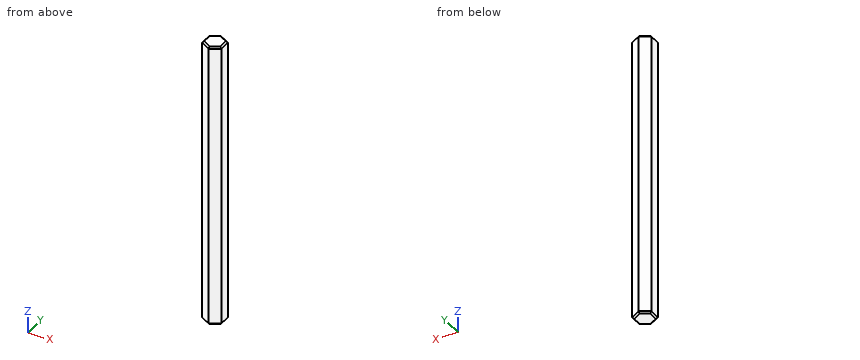
```python
from build123d import *

# Parameters (mm, degrees)
BOSS_EXTRUDE1_DEPTH = 75
CHAMFER1_SIZE       = 0.4


with BuildPart() as part:
    # Sketch1 → Boss-Extrude1 (new body)
    with BuildSketch(Plane.XY.offset(75)):
        Polygon((0, -2.886751346), (2.5, -1.443375673), (2.5, 1.443375673), (0, 2.886751346), (-2.5, 1.443375673), (-2.5, -1.443375673), align=None)
    extrude(amount=-BOSS_EXTRUDE1_DEPTH)

    # Chamfer1
    chamfer1_edges = [part.edges().sort_by_distance(p)[0] for p in [
        (2.5, 0, 0),
        (1.25, 2.165063509, 0),
        (-1.25, 2.165063509, 0),
        (-2.5, 0, 0),
        (-1.25, -2.165063509, 0),
        (-2.5, 0, 75),
        (-1.25, 2.165063509, 75),
        (1.25, 2.165063509, 75),
        (1.25, -2.165063509, 0),
        (2.5, 0, 75),
        (1.25, -2.165063509, 75),
        (-1.25, -2.165063509, 75),
    ]]
    chamfer(chamfer1_edges, length=CHAMFER1_SIZE)


solid = part.part
```
Work out the finished part from the listing and answer in its coordinate system (mm). Round coordinates to 2 decimals unless told otherwise and drop trailing zeros. Loops run counter-clockwise (first coordinate to the right, second up) from the corner with the lowest first, then second, coordinate; pieces in that order, holes last. Notation, with made-up numbers: M -28,37.25 L 14,37.25 A18 ccw 14,66.25 Z; hole C 46.5,67 d5. An arc over 180 degrees is marked long. Use CSV: the item, a comma, the result in double quotes.
Q1. Section A-A, the plane z = 23 is taken. Determine the outline of the cut face in (x, y), then the cut area to 3 significant figures.
Determined:
outline,"M -2.5,-1.44 L 0,-2.89 L 2.5,-1.44 L 2.5,1.44 L 0,2.89 L -2.5,1.44 Z"
area,"21.7 mm2"
Q2. Consider L1, parallel to Y at x = -1.35, z = 32.5; L2, parallel to X at y = -2.05, z = 65.5; L3, parallel to X at y = 1.7, z = 58. Determine where each line is inside the solid, lowest interval first.
Determined:
L1,"-2.11 to 2.11"
L2,"-1.45 to 1.45"
L3,"-2.06 to 2.06"
Q3. Section B-B, the plane x = 1.35 is taken. Determine the outline of the cut face in (y, z).
Determined:
outline,"M -2.11,0.4 L -1.65,0 L 1.65,0 L 2.11,0.4 L 2.11,74.6 L 1.65,75 L -1.65,75 L -2.11,74.6 Z"
